The listing builds one solid part. Answer for the finished solid, in the listing's coordinates (mm). Face numbers are marked on the shaded views. A direction names the side the tool comes from. Give positions to 0.01 mm unless a question says otherwise; leave off trailing zeros. Order: outer loops, then holes, each group sorted by start corner. A loop starts at its lowest first (then second) coordinate and runs counter-clockwise, first axis right, second up. Notation, with made-up numbers: (-9.5, -34) - (-2.5, -34) arc R18 cw to (-2.5, -23) - close; hole circle Ø3 at (-13.75, 87). An arc over 180 degrees is marked (long way). Use a Markdown table: item, result. Add a question column.
1) Find section B-B, the plane y = 232. Determine the outline of the cut face in (x, z), plus the area to 3 significant figures.
2) Find section D-D, the plane x = 283.5. Determine the outline of the cut face in (y, z).
3) Flat-ended cylindrical pins translate along their axes: pin 1 (10 mm diameter, centred on x = 252.5, y = 119.5, fed in from +Z); pin 2 (6 mm diameter, centred on x = 196, z = 24.5, fed in from +Y); pin 3 (3 mm diameter, centred on y = 304, z = 4, fed in from -X). Find the tip coordinate at first contact, or state that the pin passes through.
4) Straight lines are drawn through the part: line 1 (Z direction, x = 209.5, y = 175.5); line 2 (Y direction, x = 318, z = 6). For each, find the intervals that lie inside material, in ascending order.
5) For the marked faces 1 and 2, determine the directions among +Z, -Z, +X, -X, +Y, -Y from which every point of the face is accessible in a straight line to the end or side of a thin tool.
6) Find section A-A, the plane x = 325.5. Determine the outline of the cut face in (y, z).
7) Find section C-C, the plane z = 24.75. Determine the outline of the cut face in (x, y), plus the area to 3 significant figures.
Autodesk Inventor part; units mm, degrees
ref_plane "YZ Plane" through (0, 0, 0) normal (1, 0, 0) x (0, 1, 0)
ref_plane "XZ Plane" through (0, 0, 0) normal (0, 1, 0) x (-1, 0, 0)
ref_plane "XY Plane" through (0, 0, 0) normal (0, 0, 1) x (1, 0, 0)
ref_plane "Work Plane1" through (0, 0, 0) normal (0, 0, 1) x (1, 0, 0)
sketch "Sketch1" plane through (0, 0, 0) normal (0, 0, 1) x (1, 0, 0)
  arc A0 (381.5, 18.5) -> (0, 400) centre (0, 18.5) ccw
  line L0 (381.5, 18.5) -> (81.5, 18.5)
  line L1 (81.5, 18.5) -> (81.5, 391.1929)
  line L2 (81.5, 18.5) -> (381.5, 18.5)
  line L3 (381.5, 18.5) -> (381.5, -1.5)
  line L4 (381.5, -1.5) -> (81.5, -1.5)
  line L5 (81.5, -1.5) -> (81.5, 18.5)
  point P0 (0, 0)
  dimension "d0" = 300
  dimension "d2" = 20
extrude "Plate1" add sketch "Sketch1" along normal blind 1.5
sketch "Sketch2" plane through (0, 0, 1.5) normal (0, 0, 1) x (1, 0, 0)
  arc A0 (381.5, 18.5) -> (81.5, 391.1929) centre (0, 18.5) ccw
  line L0 (81.5, -1.5) -> (81.5, 391.1929)
  line L1 (381.5, -1.5) -> (81.5, -1.5)
  line L2 (381.5, 18.5) -> (381.5, -1.5)
  line L3 (81.5, 8.5) -> (381.5, 8.5)
  point P0 (0, 0)
  dimension "d3" = 10
extrude "Extrusion1" cut sketch "Sketch2" against normal through all contours L2 L1 L0 L3
sketch "Sketch3" plane through (381.5, 10, 0) normal (0, -1, 0) x (1, 0, 0)
  line L0 (-300, 0) -> (0, 0)
  line L1 (0, 0) -> (0, 30)
  line L2 (0, 30) -> (-300, 30)
  line L3 (-300, 30) -> (-300, 0)
edge flange "Flange1" height 30 angle 90 thickness 1.5 bend radius 1.5 thickness toward (0, -1, 0) relief tear relief width 1.5 relief depth 0.75 edges at (231.5, 8.5, 1.5) wall of the first edge with corners at (81.5, 10, 0) (381.5, 10, 0) (381.5, 10, 30) (81.5, 10, 30)
bend "Bend1"
corner "Corner1"
equation "\"d1\" = Thickness"
equation "\"d6\" = BendReliefWidth"
equation "\"d7\" = BendReliefDepth"
equation "\"d8\" = MinimumRemnant"
equation "\"d9\" = TransitionRadius"
equation "\"d12\" = BendRadius"
equation "\"d13\" = CornerReliefSize"
equation "\"d14\" = GapSize"
equation "\"d15\" = JacobiRadiusSize"
equation "\"BendRadius\" = Thickness"
equation "\"BendReliefWidth\" = Thickness"
equation "\"BendReliefDepth\" = 0.5 * Thickness"
equation "\"CornerReliefSize\" = 4 * Thickness"
equation "\"MinimumRemnant\" = 2 * Thickness"
equation "\"TransitionRadius\" = BendRadius"
equation "\"JacobiRadiusSize\" = BendRadius"
equation "\"GapSize\" = Thickness"
properties part number "CHAPA_7"
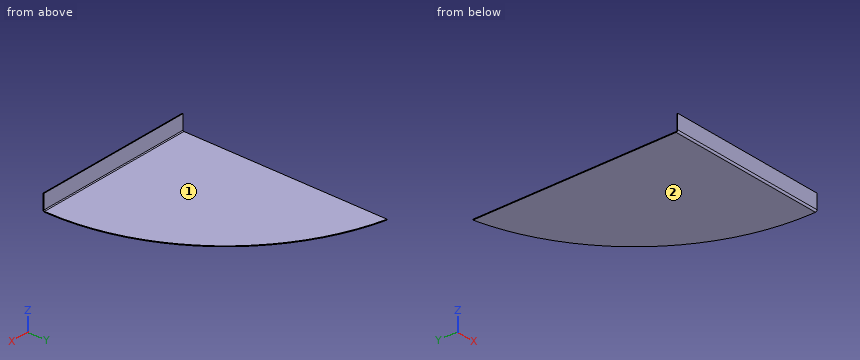
The answers:
| question | item | result |
|---|---|---|
| 1 | outline | (81.5, 0) - (316.16, 0) - (316.16, 1.5) - (81.5, 1.5) - close |
| 1 | area | 352 mm2 |
| 2 | outline | (8.5, 3) arc R3 ccw to (11.5, 0) - (273.78, 0) - (273.78, 1.5) - (11.5, 1.5) arc R1.5 cw to (10, 3) - (10, 30) - (8.5, 30) - close |
| 3 | pin 1 | z = 1.5 |
| 3 | pin 2 | y = 10 |
| 3 | pin 3 | through |
| 4 | line 1 | 0 to 1.5 |
| 4 | line 2 | 8.5 to 10 |
| 5 | face 1 | +Z, +X, -X, +Y |
| 5 | face 2 | -Z, +X, -X, +Y, -Y |
| 6 | outline | (8.5, 3) arc R3 ccw to (11.5, 0) - (217.48, 0) - (217.48, 1.5) - (11.5, 1.5) arc R1.5 cw to (10, 3) - (10, 30) - (8.5, 30) - close |
| 7 | outline | (81.5, 8.5) - (381.5, 8.5) - (381.5, 10) - (81.5, 10) - close |
| 7 | area | 450 mm2 |
